```python
from build123d import *

# Parameters (mm, degrees)
SKETCH11_W          = 24.765
SKETCH11_H          = 32.385
SKETCH11_R          = 2.032
BOSS_EXTRUDE1_DEPTH = 6.35
SKETCH12_W          = 24.765
SKETCH12_H          = 4.064
SKETCH14_W          = 24.765
SKETCH14_H          = 3.302
BOSS_EXTRUDE2_DEPTH = 28.702
CUT_EXTRUDE1_REACH  = 43.659
SKETCH15_R          = 9.017


with BuildPart() as part:
    # Sketch11 → Boss-Extrude1 (new body)
    with BuildSketch(Plane(origin=(0, 0, 0), x_dir=(1, 0, 0), z_dir=(0, 1, 0))):
        with Locations((12.3825, 16.1925)):
            Rectangle(SKETCH11_W, SKETCH11_H)
        with Locations(Location((4.7625, 27.6225, 0), (0, 0, 270))):
            Circle(SKETCH11_R, mode=Mode.SUBTRACT)
        with Locations(Location((20.0025, 27.6225, 0), (0, 0, 270))):
            Circle(SKETCH11_R, mode=Mode.SUBTRACT)
        with Locations(Location((12.3825, 6.7945, 0), (0, 0, 270))):
            Circle(SKETCH11_R, mode=Mode.SUBTRACT)
    extrude(amount=BOSS_EXTRUDE1_DEPTH)

    # Sketch12 → Cut-Revolve1 (revolve, cut)
    with BuildSketch(Plane(origin=(0, 6.35, 0), x_dir=(1, 0, 0), z_dir=(0, 1, 0))):
        with Locations((12.3825, 15.1765)):
            Rectangle(SKETCH12_W, SKETCH12_H)
    revolve(axis=Axis((0, 6.35, -17.2085), (1, 0, 0)), mode=Mode.SUBTRACT)

    # Sketch14 → Boss-Extrude2 (add)
    with BuildSketch(Plane.XZ):
        with Locations((12.3825, -16.764)):
            Rectangle(SKETCH14_W, SKETCH14_H)
    extrude(amount=BOSS_EXTRUDE2_DEPTH)

    # Sketch15 → Cut-Extrude1 (cut, up to next)
    with BuildSketch(Plane.XY.offset(-15.113), mode=Mode.PRIVATE) as cut_extrude1_sk1:
        with Locations((12.3825, -15.748)):
            Circle(SKETCH15_R)
    cut_extrude1_tool1 = extrude(cut_extrude1_sk1.sketch, amount=-CUT_EXTRUDE1_REACH, mode=Mode.PRIVATE) & part.part
    add(cut_extrude1_tool1.solids().sort_by_distance((12.3825, -15.748, -15.113))[0], mode=Mode.SUBTRACT)


solid = part.part
```
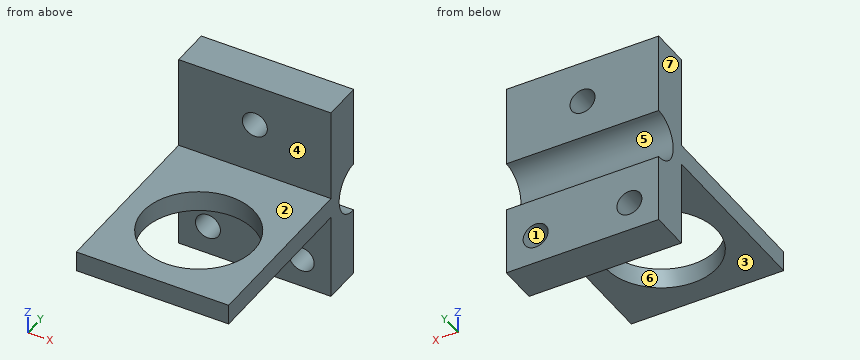
Geometry check sheet. Reference: the model listing, model coordinates, mm. Face numbers are marked on the shaded views. A direction names the side the tool comes from. Round coordinates to 2 decimals unless told otherwise and drop trailing zeros. Order: outer loops, then holes, each group sorted by start corner. A loop starts at its lowest first (then second) coordinate and runs counter-clockwise, first axis right, second up. Notation, with made-up numbers: (-32, 4.5) - (-17, 4.5) arc R21 cw to (-17, 14.5) - close; hole circle Ø3 at (-34.5, 46). An arc over 180 degrees is marked (long way). Use a Markdown table: item, result. Add a question column.
(1) Sectioned sample at C-C, the plane y = -21.5. Enter the section's corners in (x, z) (3 decimals).
(2) Material ranges on line 1 along Z through (x, y) = (4.75, 2) (3 decimals); line 2 along Z through (x, y) = (15.25, -27) (3 decimals); line 3 along Y through (x, z) = (19.5, -6.5), recorded low to high. Write a range as [from, to].
(3) Release check for a two-part mould opening along Y. For the marked faces 4, 5, 6 and 7 record: pulls with the +Y half, pulls with the -Y half, needs draft (parallel to the pull), parting line crosses it, or undercut.
(4) Sectioned sample at B-B, the plane x = 20.5. Count the separate pieces of the cut face and the enclosed holes in it, and give its area (3 significant figures).
(5) Sectioned sample at D-D, the plane z = -28. Enter the section's corners in (x, y) (3 decimals).
(6) Depth check by flat-ended pin: pin 1 (6.5 mm diameter, centred on x = 4.76, z = -27.62, fed in from -Y); pin 2 (11 mm diameter, centred on x = 12.38, y = -15.75, fed in from -Z); pin 3 (12 mm diameter, centred on x = 17, y = -23.5, fed in from +Z). Enter the tip coordinate at first touch or a pass-through.
(7) Tool access check on the marked faces 1, 2 and 3. Record the directions out of +Z, -Z, +X, -X, +Y, -Y that give a thin tool (end or side, any length) a straight path to the whole face; none if there is none.
(8) Sectioned sample at A-A, the plane y = 4. Enter the section's corners in (x, z) (1 decimal), and give its area (3 significant figures).
Answers below:
| question | item | result |
|---|---|---|
| 1 | outline | (0, -18.415) - (5.438, -18.415) - (5.438, -15.113) - (0, -15.113) - close; (19.327, -18.415) - (24.765, -18.415) - (24.765, -15.113) - (19.327, -15.113) - close |
| 2 | line 1 | [-32.385, -29.654], [-25.591, 0] |
| 2 | line 2 | [-18.415, -15.113] |
| 2 | line 3 | [0, 6.35] |
| 3 | face 4 | pulls with the -Y half |
| 3 | face 5 | pulls with the +Y half |
| 3 | face 6 | undercut |
| 3 | face 7 | needs draft |
| 4 | separate pieces | 3 |
| 4 | enclosed holes | 0 |
| 4 | area | 224 mm² |
| 5 | outline | (0, 0) - (2.766, 0) - (2.766, 6.35) - (0, 6.35) - close; (6.759, 0) - (18.006, 0) - (18.006, 6.35) - (6.759, 6.35) - close; (21.999, 0) - (24.765, 0) - (24.765, 6.35) - (21.999, 6.35) - close |
| 6 | pin 1 | y = 0 |
| 6 | pin 2 | through |
| 6 | pin 3 | z = -15.11 |
| 7 | face 1 | +Y, -Y |
| 7 | face 2 | +Z, +X, -X, -Y |
| 7 | face 3 | -Z, +X, -X, -Y |
| 8 | outline | (0, -32.4) - (24.8, -32.4) - (24.8, -20.5) - (0, -20.5) - close; (0, -13.9) - (24.8, -13.9) - (24.8, 0) - (0, 0) - close; hole circle Ø4.1 at (4.8, -27.6); hole circle Ø4.1 at (12.4, -6.8); hole circle Ø4.1 at (20, -27.6) |
| 8 | area | 599 mm² |
